from build123d import *

# Parameters (mm, degrees)
SKETCH1_R           = 5
BOSS_EXTRUDE1_DEPTH = 12.7
FILLET1_R           = 1.27


with BuildPart() as part:
    # Sketch1 → Boss-Extrude1 (new body, symmetric)
    with BuildSketch(Plane.XY):
        Polygon((-19.05, 0), (19.05, 0), (19.05, 9.525), (9.525, 9.525), (9.525, 19.05), (-9.525, 19.05), (-9.525, 9.525), (-19.05, 9.525), align=None)
        with Locations((0, 10.764499551)):
            Circle(SKETCH1_R, mode=Mode.SUBTRACT)
    extrude(amount=BOSS_EXTRUDE1_DEPTH, both=True)

    # Fillet1
    fillet1_edges = [part.edges().sort_by_distance(p)[0] for p in [
        (-9.525, 9.525, 0),
        (9.525, 9.525, 0),
    ]]
    fillet(fillet1_edges, radius=FILLET1_R)


solid = part.part
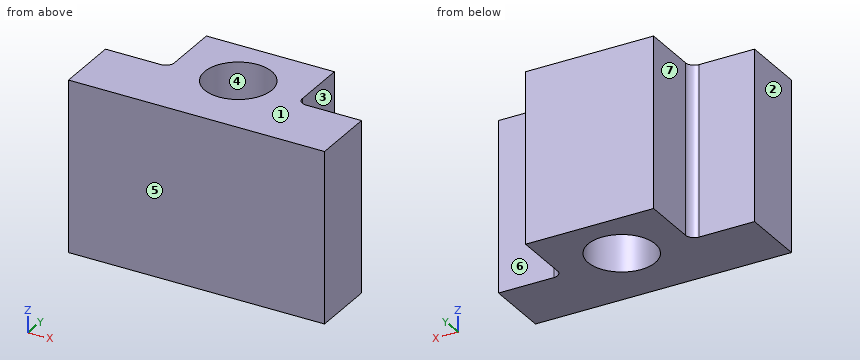
Input: part model. Units: mm. Frame: model coordinates. Face numbers are marked on the shaded views. A direction names the side the tool comes from. Round coordinates to 2 decimals unless told otherwise and drop trailing zeros. Loops run counter-clockwise (first coordinate to the right, second up) from the corner with the lowest first, then second, coordinate; pieces in that order, holes last. Notation, with made-up numbers: (-15, 6.25) -> (-3, 6.25) arc R15 cw to (-3, 30.25) -> close; hole circle Ø10 at (59.5, 26.25). An arc over 180 degrees is marked (long way). Answer as a JSON object with one key per item and string values. Group by question number.
1) Section query A-A on x = 0. Output: boundary loops of the cut face in (y, z).
2) Reachability of the marked faces 5, 6 and 7 from +Z, -Z, +X, -X, +Y, -Y: full face, straight path, thin tool, end or side. Return the list, or none.
3) Ray query, L1, parallel to X at y = 10.75, z = 10.5; L2, parallel to Y at x = 0, z = -7; L3, parallel to X at y = 13, z = 9.75 (3 decimals). Return the intervals inside material, ascending.
4) Pin query (flat end, axial travel): pin 1 (9 mm diameter, centred on y = 15.5, z = -5, fed in from +X) (3 decimals); pin 2 (2.5 mm diameter, centred on y = 15, z = 5.5, fed in from -X) (3 decimals); pin 3 (6.5 mm diameter, centred on x = -14.5, z = 4.5, fed in from +Y) (3 decimals); pin 4 (3 mm diameter, centred on x = -0.5, y = 8.5, fed in from -Z). Return the tip coordinate at first contact, or that it passes through.
5) Draft query along X for the marked faces 1, 2, 3 and 4. Return one class per face: +X half, -X half, draft (parallel to the pull), parting line (faces both ways), or undercut.
6) Section query B-B on y = 12. Output: boundary loops of the cut face in (x, z) (3 decimals), plus the area to 3 significant figures.
7) Section query D-D on x = 14. Output: boundary loops of the cut face in (y, z) (3 decimals).
Reply:
{
 "1": {"outline": "(0, -12.7) -> (5.76, -12.7) -> (5.76, 12.7) -> (0, 12.7) -> close; (15.76, -12.7) -> (19.05, -12.7) -> (19.05, 12.7) -> (15.76, 12.7) -> close"},
 "2": {"face 5": "+Z, -Z, +X, -X, -Y", "face 6": "+Z, -Z, +X, +Y", "face 7": "+Z, -Z, -X, +Y"},
 "3": {"L1": "x = -9.53 to -5, 5 to 9.53", "L2": "y = 0 to 5.76, 15.76 to 19.05", "L3": "x = -9.525 to -4.472, 4.472 to 9.525"},
 "4": {"pin 1": "stops at x = 9.525", "pin 2": "stops at x = -9.525", "pin 3": "stops at y = 9.525", "pin 4": "passes through"},
 "5": {"face 1": "draft", "face 2": "-X half", "face 3": "+X half", "face 4": "undercut"},
 "6": {"outline": "(-9.525, -12.7) -> (-4.845, -12.7) -> (-4.845, 12.7) -> (-9.525, 12.7) -> close; (4.845, -12.7) -> (9.525, -12.7) -> (9.525, 12.7) -> (4.845, 12.7) -> close", "area": "238 mm2"},
 "7": {"outline": "(0, -12.7) -> (9.525, -12.7) -> (9.525, 12.7) -> (0, 12.7) -> close"}
}
